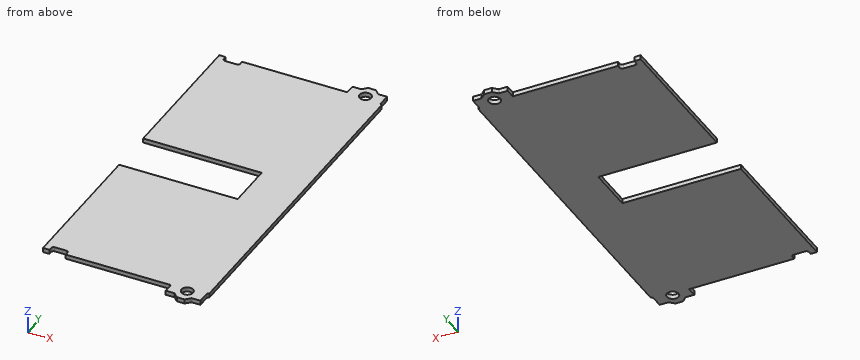
```python
from build123d import *

# Parameters (mm, degrees)
SKETCH1_R           = 5
BOSS_EXTRUDE1_DEPTH = 3.8


with BuildPart() as part:
    # Sketch1 → Boss-Extrude1 (new body)
    with BuildSketch(Plane.XY):
        with BuildLine():
            Line((-124.434769571, -238.739800618), (-118.934676066, -238.739800618))
            Line((-118.934676066, -238.739800618), (-118.934676066, -235.848726439))
            ThreePointArc((-118.934676066, -235.848726439), (-118.348889629, -234.434512877), (-116.934676066, -233.848726439))
            Line((-116.934676066, -233.848726439), (-106.934769571, -233.848726439))
            ThreePointArc((-106.934769571, -233.848726439), (-105.520556009, -234.434512877), (-104.934769571, -235.848726439))
            Line((-104.934769571, -235.848726439), (-104.934769571, -238.848726439))
            Line((-104.934769571, -238.848726439), (-14.85, -238.848726439))
            Line((-14.85, -238.848726439), (-14.85, -247.348726439))
            Line((-14.85, -247.348726439), (-7.707106781, -247.348726439))
            ThreePointArc((-7.707106781, -247.348726439), (-7.324423349, -247.424846907), (-7, -247.641619658))
            Line((-7, -247.641619658), (-3.292893219, -251.348726439))
            Line((-3.292893219, -251.348726439), (3.292893219, -251.348726439))
            Line((3.292893219, -251.348726439), (7, -247.641619658))
            ThreePointArc((7, -247.641619658), (7.324423349, -247.424846907), (7.707106781, -247.348726439))
            Line((7.707106781, -247.348726439), (14.85, -247.348726439))
            Line((14.85, -247.348726439), (14.85, -237.15583322))
            ThreePointArc((14.85, -237.15583322), (14.926120467, -236.773149788), (15.142893219, -236.448726439))
            Line((15.142893219, -236.448726439), (16.4, -235.191619658))
            Line((16.4, -235.191619658), (16.4, 50.89416678))
            Line((16.4, 50.89416678), (15.142893219, 52.151273561))
            ThreePointArc((15.142893219, 52.151273561), (14.926120467, 52.47569691), (14.85, 52.858380342))
            Line((14.85, 52.858380342), (14.85, 63.051273561))
            Line((14.85, 63.051273561), (7.707106781, 63.051273561))
            ThreePointArc((7.707106781, 63.051273561), (7.324423349, 63.127394028), (7, 63.34416678))
            Line((7, 63.34416678), (3.292893219, 67.051273561))
            Line((3.292893219, 67.051273561), (-3.292893219, 67.051273561))
            Line((-3.292893219, 67.051273561), (-7, 63.34416678))
            ThreePointArc((-7, 63.34416678), (-7.324423349, 63.127394028), (-7.707106781, 63.051273561))
            Line((-7.707106781, 63.051273561), (-14.85, 63.051273561))
            Line((-14.85, 63.051273561), (-14.85, 54.551273561))
            Line((-14.85, 54.551273561), (-104.934769571, 54.551273561))
            Line((-104.934769571, 54.551273561), (-104.934769571, 51.551273561))
            ThreePointArc((-104.934769571, 51.551273561), (-105.520556009, 50.137059998), (-106.934769571, 49.551273561))
            Line((-106.934769571, 49.551273561), (-116.934769571, 49.551273561))
            ThreePointArc((-116.934769571, 49.551273561), (-118.348983134, 50.137059998), (-118.934769571, 51.551273561))
            Line((-118.934769571, 51.551273561), (-118.934769571, 54.551273561))
            Line((-118.934769571, 54.551273561), (-124.434769571, 54.551273561))
            Line((-124.434769571, 54.551273561), (-124.434769571, -72.148726439))
            Line((-124.434769571, -72.148726439), (-22.877938229, -72.148726439))
            Line((-22.877938229, -72.148726439), (-22.877938229, -112.148726439))
            Line((-22.877938229, -112.148726439), (-124.434769571, -112.148726439))
            Line((-124.434769571, -112.148726439), (-124.434769571, -238.739800618))
        make_face()
        with Locations(Location((0, -240.335275852, 0), (0, 0, 180))):
            Circle(SKETCH1_R, mode=Mode.SUBTRACT)
        with Locations(Location((0, 56.037822974, 0), (0, 0, 180))):
            Circle(SKETCH1_R, mode=Mode.SUBTRACT)
    extrude(amount=BOSS_EXTRUDE1_DEPTH)


solid = part.part
```
Design review of the part built by this model. Coordinates are the model's own, in mm. Give positions to 0.01 mm unless a question says otherwise; leave off trailing zeros. Order: outer loops, then holes, each group sorted by start corner. A loop starts at its lowest first (then second) coordinate and runs counter-clockwise, first axis right, second up. Notation, with made-up numbers: (86.5, 26) - (98.5, 26) arc R15 cw to (98.5, 37) - close; hole circle Ø6 at (6, 15). An arc over 180 degrees is marked (long way). Use a Markdown table: item, result. Add a question column.
(1) Wall thickness on probe 1 along Y at (x, z) = (0, 2.35); probe 2 along Y at (x, z) = (-40.5, 0.9); probe 3 along Y at (x, z) = (-115, 3): over which ranges is each line inside the solid? List them lowest first. Write a range as [from, to].
(2) Add section B-B on z = 1.15. Give the number of separate pieces and of enclosed holes in the cut face, then the cut area to 3 significant figures.
(3) Add section A-A on x = 0. Give the boundary of the cut face in (y, z), then the cut area to 3 significant figures.
(4) Clearance check with flat-ended pins moving along their axes: P1, Ø1.9, axis at x = 11, z = 1, coming from the -Y side; P2, Ø1.9, axis at x = -79.5, z = 3, coming from the +Y side; P3, Ø1.1, axis at x = -121, z = 2.5, coming from the -Y side. State where each tip first meets the part, or that it passes through.
Report:
| question | item | result |
|---|---|---|
| 1 | probe 1 | y = [-251.35, -245.34], [-235.34, 51.04], [61.04, 67.05] |
| 1 | probe 2 | y = [-238.85, -112.15], [-72.15, 54.55] |
| 1 | probe 3 | y = [-233.85, -112.15], [-72.15, 49.55] |
| 2 | separate pieces | 1 |
| 2 | enclosed holes | 2 |
| 2 | area | 37,500 mm² |
| 3 | outline | (-251.35, 0) - (-245.34, 0) - (-245.34, 3.8) - (-251.35, 3.8) - close; (-235.34, 0) - (51.04, 0) - (51.04, 3.8) - (-235.34, 3.8) - close; (61.04, 0) - (67.05, 0) - (67.05, 3.8) - (61.04, 3.8) - close |
| 3 | area | 1,130 mm² |
| 4 | P1 | stops at y = -247.35 |
| 4 | P2 | stops at y = 54.55 |
| 4 | P3 | stops at y = -238.74 |
